Autodesk Inventor part; units mm, degrees
ref_plane "Work Plane1" through (0, -14.5, 0) normal (0, 1, 0) x (-1, 0, 0)
ref_plane "Work Plane2" through (0, 14.5, 0) normal (0, 1, 0) x (-1, 0, 0)
ref_plane "YZ Plane" through (0, 0, 0) normal (1, 0, 0) x (0, 1, 0)
sketch "Sketch2" plane through (0, 0, 0) normal (0, 1, 0) x (-1, 0, 0)
  circle A0 centre (-25, -75) radius 36 construction
  line L0 (-25, -75) -> (-61, -75) construction
  line L1 (-25, -75) -> (4.6941, -54.6466) construction
  circle A1 centre (-25, -75) radius 41.5
  circle A2 centre (-25, -75) radius 28
  arc A3 (-8.1325, -52.6508) -> (0, -41.8752) centre (-4.0663, -47.263) ccw
  arc A4 (-50, -41.8752) -> (-39.3017, -48.5193) centre (-45.9337, -47.263) ccw
  line L2 (-25, -75) -> (-4.0663, -47.263) construction
  circle A5 centre (-25, -75) radius 31.5
  line L3 (0, -41.8752) -> (0, 0)
  line L4 (-50, -41.8752) -> (-50, 0)
  line L5 (0, 0) -> (-50, 0)
  line L6 (-25, 0) -> (-25, -75) construction
  point P0 (15.9829, -68.469)
  point P1 (13.8342, -60.366)
  point P2 (-39.2078, -46.6936)
  point P3 (-41.8675, -52.6508)
  point P4 (-8.1325, -52.6508)
  dimension "d1" = 72
  dimension "d5" = 83
  dimension "d6" = 56
  dimension "d7" = 63
  dimension "d11" = 50
  dimension "d31" = 75
ref_plane "Work Plane1" through (0, -14.5, 0) normal (0, 1, 0) x (-1, 0, 0)
ref_plane "Work Plane2" through (0, 14.5, 0) normal (0, 1, 0) x (-1, 0, 0)
extrude "Extrusion1" add sketch "Sketch2" along normal blind 12 from surface at 14.5 contours A1 A4 A5 A3 | A3 A5 A4 A1
extrude "Extrusion2" add sketch "Sketch2" against normal blind 12 from surface at -14.5 contours A3 A5 A4 A1 | A3 A2 A4 A5 picked at (-44.9519, -42.6635) picked at (-38.3765, -47.944)
extrude "Extrusion3" add sketch "Sketch2" along normal mid plane 53 contours A1 L4 L5 L3
sketch "Sketch3" plane through (0, 0, 0) normal (1, 0, 0) x (0, 1, 0)
  line L0 (-26.5, 0) -> (26.5, 0)
  circle A0 centre (0, 0) radius 26.5
extrude "Extrusion4" add sketch "Sketch3" along normal up to surface (50 mm away)
properties part number "hip_back_left"
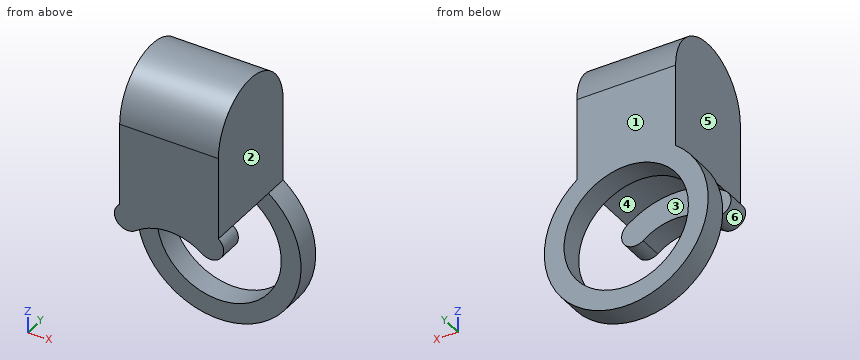
Source: CAD feature listing. Evaluate the final solid. Frame: model axes, mm. Face numbers are marked on the shaded views. A direction names the side the tool comes from. Round coordinates to 2 decimals unless told otherwise and drop trailing zeros. Loops run counter-clockwise (first coordinate to the right, second up) from the corner with the lowest first, then second, coordinate; pieces in that order, holes last.
1. Section query C-C on z = -102. Output: boundary loops of the cut face in (x, y).
2. Ray query, L1, parallel to X at y = 21.5, z = -75; L2, parallel to Z at x = 25, y = 21; L3, parallel to Y at x = 61, z = -58.5. Return the intervals inside material, ascending.
3. Contact query for flat-ended pins moving along their axis: pin 1 (2 mm diameter, centred on x = 5, y = 16.5, fed in from +Z); pin 2 (12 mm diameter, centred on x = 52.5, y = 18.5, fed in from +Z); pin 3 (16 mm diameter, centred on y = -10.5, z = 9, fed in from -X). Output: stop coordinate, or through.
4. Section query B-B on x = 13. Output: boundary loops of the cut face in (y, z), and give its area (3 significant figures).
5. Mould query, pull axis X, two halves, no side actions, for the marked faces 1, 2 and 3. Classes: released by +X, released by -X, zero draft, split by the parting line, or undercut.
6. Section query D-D on y = -17.5. Output: boundary loops of the cut face in (x, z), and give its area (3 significant figures).
7. Access query for the marked faces 4, 5 and 6. Directions: +Z, -Z, +X, -X, +Y, -Y. A direction counts if a zero-diameter tool reaches every point of the face in a straight line with its end or side. Return the directions, or none.
8. Section query A-A on z = -75. Output: boundary loops of the cut face in (x, y).
Answers below:
1. outline: (-6.52, 14.5) - (8.78, 14.5) - (8.78, 26.5) - (-6.52, 26.5) - close; (41.22, 14.5) - (56.52, 14.5) - (56.52, 26.5) - (41.22, 26.5) - close
2. L1: x = -16.5 to -6.5, 56.5 to 66.5
2. L2: z = -116.5 to -106.5, -43.5 to 16.16
2. L3: y = 14.5 to 26.5
3. pin 1: stops at z = 21.49
3. pin 2: stops at z = 23.07
3. pin 3: stops at x = 0
4. outline: (-26.5, -49.7) - (-14.5, -49.7) - (-14.5, -35.27) - (14.5, -35.27) - (14.5, -45.88) - (26.5, -45.88) - (26.5, 0) arc R26.5 ccw to (-26.5, 0) - close; (14.5, -114.73) - (26.5, -114.73) - (26.5, -104.12) - (14.5, -104.12) - close
4. area: 3,400 mm2
5. face 1: zero draft
5. face 2: released by +X
5. face 3: undercut
6. outline: (0, -41.88) arc R6.75 ccw to (8.13, -52.65) arc R28 cw to (41.87, -52.65) arc R6.75 ccw to (50, -41.88) - (50, 19.9) - (0, 19.9) - close
6. area: 3,550 mm2
7. face 4: -Z
7. face 5: +Z, -X, +Y, -Y
7. face 6: -Y
8. outline: (-16.5, 14.5) - (-6.5, 14.5) - (-6.5, 26.5) - (-16.5, 26.5) - close; (56.5, 14.5) - (66.5, 14.5) - (66.5, 26.5) - (56.5, 26.5) - close
